from build123d import *

# Parameters (mm, degrees)
SKETCH1_W           = 30
SKETCH1_H           = 35
BOSS_EXTRUDE1_DEPTH = 60
SKETCH2_R           = 8
CUT_EXTRUDE1_DEPTH  = 76.663729752
SKETCH3_R           = 5
CUT_EXTRUDE2_DEPTH  = 10
SKETCH5_R           = 2.5
CUT_EXTRUDE4_DEPTH  = 15


with BuildPart() as part:
    # Sketch1 → Boss-Extrude1 (new body)
    with BuildSketch(Plane.XY):
        with Locations((15, 17.5)):
            Rectangle(SKETCH1_W, SKETCH1_H)
    extrude(amount=BOSS_EXTRUDE1_DEPTH)

    # Sketch2 → Cut-Extrude1 (cut, through all)
    with BuildSketch(Plane(origin=(30, 0, 0), x_dir=(0, 0, -1), z_dir=(1, 0, 0))):
        with Locations(Location((-45, 17.5, 0), (0, 0, 90))):
            Circle(SKETCH2_R)
    extrude(amount=-CUT_EXTRUDE1_DEPTH, mode=Mode.SUBTRACT)

    # Sketch3 → Cut-Extrude2 (cut)
    with BuildSketch(Plane(origin=(0, 0, 0), x_dir=(-1, 0, 0), z_dir=(0, 0, -1))):
        with Locations((-15, 17.5)):
            Circle(SKETCH3_R)
    extrude(amount=-CUT_EXTRUDE2_DEPTH, mode=Mode.SUBTRACT)

    # Sketch5 → Cut-Extrude4 (cut)
    with BuildSketch(Plane(origin=(0, 35, 0), x_dir=(1, 0, 0), z_dir=(0, 1, 0))):
        with Locations(Location((15, -5, 0), (0, 0, 270))):
            Circle(SKETCH5_R)
    extrude(amount=-CUT_EXTRUDE4_DEPTH, mode=Mode.SUBTRACT)


solid = part.part
CAD build for the part. Positions are in the model's coordinates, mm. A direction names the side the tool comes from. Give positions to 0.01 mm unless a question says otherwise; leave off trailing zeros. Order: outer loops, then holes, each group sorted by start corner. A loop starts at its lowest first (then second) coordinate and runs counter-clockwise, first axis right, second up. Notation, with made-up numbers: (-32, 82.5) - (24, 82.5) arc R22 cw to (24, 97.5) - close; hole circle Ø5 at (-36, 75). An arc over 180 degrees is marked (long way). Answer in a Markdown table with one row per item.
1. Tool access for faces 4 (the flat face through (30, 17, 30)), 5 (the cylindrical face through (12.78, 28.51, 6.15)), 6 (the cylindrical face through (12.693, 13.064, 4.93)): list every direction of +Z, -Z, +X, -X, +Y, -Y with a clear straight run to the whole face (end or side of a thin tool).
Data:
| item | result |
|---|---|
| face 4 | +Z, -Z, +X, +Y, -Y |
| face 5 | +Y |
| face 6 | -Z |
2. Saw through at D-D, the plane x = 26. Give the cut face in (y, z).
Data:
| item | result |
|---|---|
| outline | (0, 0) - (35, 0) - (35, 60) - (0, 60) - close; hole circle Ø16 at (17.5, 45) |
3. Saw through at B-B, the plane x = 15. Give the cut face in (y, z), plus the area to 3 significant figures.
Data:
| item | result |
|---|---|
| outline | (0, 0) - (12.5, 0) - (12.5, 10) - (22.5, 10) - (22.5, 7.5) - (35, 7.5) - (35, 60) - (0, 60) - close; (22.5, 0) - (35, 0) - (35, 2.5) - (22.5, 2.5) - close; hole circle Ø16 at (17.5, 45) |
| area | 1,740 mm² |
4. Probe probe 1 along Z at (x, y) = (15, 30.75); probe 2 along Z at (x, y) = (22, 17.5); probe 3 along Z at (x, y) = (12.75, 24). List the from-to ranges inside material, lowest first. Write a range as [from, to].
Data:
| item | result |
|---|---|
| probe 1 | z = [0, 2.5], [7.5, 60] |
| probe 2 | z = [0, 37], [53, 60] |
| probe 3 | z = [0, 3.91], [6.09, 40.34], [49.66, 60] |
5. Saw through at A-A, the plane z = 45. Give the cut face in (x, y), plus the area to 3 significant figures.
Data:
| item | result |
|---|---|
| outline | (0, 0) - (30, 0) - (30, 9.5) - (0, 9.5) - close; (0, 25.5) - (30, 25.5) - (30, 35) - (0, 35) - close |
| area | 570 mm² |
6. Pull direction X, two halves, no side cores. Call faces 1 (the flat face through (0, 17, 30)), 2 (the flat face through (11, 22, 0)), 3 (the flat face through (15, 18, 10)): pulls with the +X half, pulls with the -X half, needs draft (parallel to the pull), parting line crosses it, or undercut.
Data:
| item | result |
|---|---|
| face 1 | pulls with the -X half |
| face 2 | needs draft |
| face 3 | undercut |
7. Flat gauge pins, fed straight in: pin 1 (3 mm diameter, centred on x = 16, y = 16.5, fed in from -Z); pin 2 (10 mm diameter, centred on x = 3.5, y = 6.5, fed in from -Z); pin 3 (9.5 mm diameter, centred on y = 17.5, z = 45, fed in from +X). Where does each tip first touch, or does it go through?
Data:
| item | result |
|---|---|
| pin 1 | stops at z = 10 |
| pin 2 | stops at z = 0 |
| pin 3 | passes through |
8. Saw through at C-C, the plane y = 17.5. Give the cut face in (x, z), plus the area to 3 significant figures.
Data:
| item | result |
|---|---|
| outline | (0, 0) - (10, 0) - (10, 10) - (20, 10) - (20, 0) - (30, 0) - (30, 37) - (0, 37) - close; (0, 53) - (30, 53) - (30, 60) - (0, 60) - close |
| area | 1,220 mm² |
